```python
from build123d import *

# Parameters (mm, degrees)
SKETCH_1_W               = 100
SKETCH_1_H               = 130
SKETCH_1_R               = 2
EXTRUDE_1_DEPTH          = 2
SKETCH_3_W               = 100
SKETCH_3_H               = 2
EXTRUDE_2_DEPTH          = 45
SKETCH_4_W               = 1.5
SKETCH_4_H               = 110
EXTRUDE_3_DEPTH          = 5
SKETCH_5_W               = 114
SKETCH_5_H               = 47
EXTRUDE_7_DEPTH          = 2
CUT_EXTRUDE_3_DEPTH      = 171.073513517
CUT_EXTRUDE_3_DEPTH_BACK = 171.073513517
EXTRUDE_10_DEPTH         = 1.5
EXTRUDE_11_DEPTH         = 114
CUT_EXTRUDE_4_REACH      = 160.267
SKETCH_13_R              = 2
SKETCH_14_R              = 10
EXTRUDE_12_DEPTH         = 22
CUT_EXTRUDE_5_REACH      = 160.267
SKETCH_15_R              = 1.5
CUT_EXTRUDE_6_REACH      = 176.781
SKETCH_16_R              = 1.5
CUT_EXTRUDE_7_REACH      = 184.153
SKETCH_17_W              = 25
SKETCH_17_H              = 35
CUT_EXTRUDE_8_REACH      = 160.267
SKETCH_18_W              = 20
SKETCH_18_H              = 30
CUT_EXTRUDE_9_REACH      = 176.781
SKETCH_19_W              = 20
SKETCH_19_H              = 28
SKETCH_19_W_2            = 15
CUT_EXTRUDE_10_REACH     = 176.781
SKETCH_20_R              = 3


with BuildPart() as part:
    # 草图1 → 凸台-拉伸1 (new body)
    with BuildSketch(Plane(origin=(0, 0, 0), x_dir=(1, 0, 0), z_dir=(0, 1, 0))):
        with Locations((50, 65)):
            Rectangle(SKETCH_1_W, SKETCH_1_H)
        with Locations(Location((15, 105, 0), (0, 0, 270))):
            Circle(SKETCH_1_R, mode=Mode.SUBTRACT)
        with Locations(Location((15, 19, 0), (0, 0, 270))):
            Circle(SKETCH_1_R, mode=Mode.SUBTRACT)
        with Locations(Location((73, 105, 0), (0, 0, 270))):
            Circle(SKETCH_1_R, mode=Mode.SUBTRACT)
        with Locations(Location((73, 19, 0), (0, 0, 270))):
            Circle(SKETCH_1_R, mode=Mode.SUBTRACT)
    extrude(amount=EXTRUDE_1_DEPTH)

    # 草图3 → 凸台-拉伸2 (add)
    with BuildSketch(Plane(origin=(0, 2, 0), x_dir=(1, 0, 0), z_dir=(0, 1, 0))):
        with Locations((50, 121)):
            Rectangle(SKETCH_3_W, SKETCH_3_H)
        with Locations((50, 9)):
            Rectangle(SKETCH_3_W, SKETCH_3_H)
    extrude(amount=EXTRUDE_2_DEPTH)

    # 草图4 → 凸台-拉伸3 (add)
    with BuildSketch(Plane(origin=(0, 2, 0), x_dir=(1, 0, 0), z_dir=(0, 1, 0))):
        with Locations((91.25, 65)):
            Rectangle(SKETCH_4_W, SKETCH_4_H)
    extrude(amount=EXTRUDE_3_DEPTH)

    # 草图5 → 凸台-拉伸7 (add)
    with BuildSketch(Plane.ZY):
        with Locations((-65, 23.5)):
            Rectangle(SKETCH_5_W, SKETCH_5_H)
    extrude(amount=EXTRUDE_7_DEPTH)

    # 草图6 → 切除-拉伸3 (cut, two sides: drawn at the far end of the back side and taken through both)
    with BuildSketch(Plane(origin=(0, 2, 0), x_dir=(1, 0, 0), z_dir=(0, 1, 0)).offset(-CUT_EXTRUDE_3_DEPTH_BACK)):
        Polygon((0, 8), (92, 8), (92, 122), (0, 122), (0, 130), (100, 130), (100, 117), (100, 13), (100, 0), (0, 0), align=None)
    extrude(amount=CUT_EXTRUDE_3_DEPTH + CUT_EXTRUDE_3_DEPTH_BACK, mode=Mode.SUBTRACT)

    # 草图11 → 凸台-拉伸10 (add)
    with BuildSketch(Plane(origin=(92, 0, 0), x_dir=(0, 0, -1), z_dir=(1, 0, 0))):
        Polygon((8, 47), (122, 47), (122, 42), (122, 0), (110, 0), (110, 37), (16, 37), (16, 0), (8, 0), align=None)
    extrude(amount=-EXTRUDE_10_DEPTH)

    # 草图12 → 凸台-拉伸11 (add, through all)
    with BuildSketch(Plane.XY.offset(-8)):
        with BuildLine():
            Line((91, 47), (91, 48.5))
            ThreePointArc((91, 48.5), (90, 51.796662955), (89, 48.5))
            Line((89, 48.5), (89, 47))
            Line((89, 47), (86, 47))
            Line((86, 47), (86, 45))
            Line((86, 45), (90, 45))
            Line((90, 45), (90, 42.318790087))
            Line((90, 42.318790087), (92, 42.318790087))
            Line((92, 42.318790087), (92, 44))
            Line((92, 44), (93.5, 44))
            ThreePointArc((93.5, 44), (96.796662955, 45), (93.5, 46))
            Line((93.5, 46), (92, 46))
            Line((92, 46), (92, 47))
            Line((92, 47), (91, 47))
        make_face()
        with BuildLine():
            Line((0, 42.318790087), (0, 45))
            Line((0, 45), (4, 45))
            Line((4, 45), (4, 47))
            Line((4, 47), (1, 47))
            Line((1, 47), (1, 48.5))
            ThreePointArc((1, 48.5), (0, 51.796662955), (-1, 48.5))
            Line((-1, 48.5), (-1, 47))
            Line((-1, 47), (-2, 47))
            Line((-2, 47), (-2, 46))
            Line((-2, 46), (-3.5, 46))
            ThreePointArc((-3.5, 46), (-6.796662955, 45), (-3.5, 44))
            Line((-3.5, 44), (-2, 44))
            Line((-2, 44), (-2, 42.318790087))
            Line((-2, 42.318790087), (0, 42.318790087))
        make_face()
        with BuildLine():
            Line((-1, 0), (-1, -1.5))
            ThreePointArc((-1, -1.5), (0, -4.796662955), (1, -1.5))
            Line((1, -1.5), (1, 0))
            Line((1, 0), (4, 0))
            Line((4, 0), (4, 2))
            Line((4, 2), (0, 2))
            Line((0, 2), (0, 4.681209913))
            Line((0, 4.681209913), (-2, 4.681209913))
            Line((-2, 4.681209913), (-2, 3))
            Line((-2, 3), (-3.5, 3))
            ThreePointArc((-3.5, 3), (-6.796662955, 2), (-3.5, 1))
            Line((-3.5, 1), (-2, 1))
            Line((-2, 1), (-2, 0))
            Line((-2, 0), (-1, 0))
        make_face()
        with BuildLine():
            Line((90, 4.681209913), (90, 2))
            Line((90, 2), (86, 2))
            Line((86, 2), (86, 0))
            Line((86, 0), (89, 0))
            Line((89, 0), (89, -1.5))
            ThreePointArc((89, -1.5), (90, -4.796662955), (91, -1.5))
            Line((91, -1.5), (91, 0))
            Line((91, 0), (92, 0))
            Line((92, 0), (92, 1))
            Line((92, 1), (93.5, 1))
            ThreePointArc((93.5, 1), (96.796662955, 2), (93.5, 3))
            Line((93.5, 3), (92, 3))
            Line((92, 3), (92, 4.681209913))
            Line((92, 4.681209913), (90, 4.681209913))
        make_face()
    extrude(amount=-EXTRUDE_11_DEPTH)

    # 草图13 → 切除-拉伸4 (cut, up to next)
    with BuildSketch(Plane.XY.offset(-8), mode=Mode.PRIVATE) as cut_extrude_4_sk1:
        with Locations((86, 40.599475321)):
            Circle(SKETCH_13_R)
    cut_extrude_4_tool1 = extrude(cut_extrude_4_sk1.sketch, amount=-CUT_EXTRUDE_4_REACH, mode=Mode.PRIVATE) & part.part
    # 草图13 → 切除-拉伸4 (cut, up to next)
    with BuildSketch(Plane.XY.offset(-8), mode=Mode.PRIVATE) as cut_extrude_4_sk2:
        with Locations((86, 5.599475321)):
            Circle(SKETCH_13_R)
    cut_extrude_4_tool2 = extrude(cut_extrude_4_sk2.sketch, amount=-CUT_EXTRUDE_4_REACH, mode=Mode.PRIVATE) & part.part
    # 草图13 → 切除-拉伸4 (cut, up to next)
    with BuildSketch(Plane.XY.offset(-8), mode=Mode.PRIVATE) as cut_extrude_4_sk3:
        with Locations((4, 5.599475321)):
            Circle(SKETCH_13_R)
    cut_extrude_4_tool3 = extrude(cut_extrude_4_sk3.sketch, amount=-CUT_EXTRUDE_4_REACH, mode=Mode.PRIVATE) & part.part
    # 草图13 → 切除-拉伸4 (cut, up to next)
    with BuildSketch(Plane.XY.offset(-8), mode=Mode.PRIVATE) as cut_extrude_4_sk4:
        with Locations((4, 40.599475321)):
            Circle(SKETCH_13_R)
    cut_extrude_4_tool4 = extrude(cut_extrude_4_sk4.sketch, amount=-CUT_EXTRUDE_4_REACH, mode=Mode.PRIVATE) & part.part
    add(cut_extrude_4_tool1.solids().sort_by_distance((86, 40.599475, -8))[0], mode=Mode.SUBTRACT)
    add(cut_extrude_4_tool2.solids().sort_by_distance((86, 5.599475, -8))[0], mode=Mode.SUBTRACT)
    add(cut_extrude_4_tool3.solids().sort_by_distance((4, 5.599475, -8))[0], mode=Mode.SUBTRACT)
    add(cut_extrude_4_tool4.solids().sort_by_distance((4, 40.599475, -8))[0], mode=Mode.SUBTRACT)

    # 草图14 → 凸台-拉伸12 (add)
    with BuildSketch(Plane(origin=(0, 0, -122), x_dir=(-1, 0, 0), z_dir=(0, 0, -1))):
        with Locations(Location((-45, 23.5, 0), (0, 0, 180))):
            Circle(SKETCH_14_R)
    extrude(amount=EXTRUDE_12_DEPTH)

    # 草图15 → 切除-拉伸5 (cut, up to next)
    with BuildSketch(Plane(origin=(0, 0, -122), x_dir=(-1, 0, 0), z_dir=(0, 0, -1)), mode=Mode.PRIVATE) as cut_extrude_5_sk1:
        with Locations((-62, 32)):
            Circle(SKETCH_15_R)
    cut_extrude_5_tool1 = extrude(cut_extrude_5_sk1.sketch, amount=-CUT_EXTRUDE_5_REACH, mode=Mode.PRIVATE) & part.part
    # 草图15 → 切除-拉伸5 (cut, up to next)
    with BuildSketch(Plane(origin=(0, 0, -122), x_dir=(-1, 0, 0), z_dir=(0, 0, -1)), mode=Mode.PRIVATE) as cut_extrude_5_sk2:
        with Locations((-62, 15)):
            Circle(SKETCH_15_R)
    cut_extrude_5_tool2 = extrude(cut_extrude_5_sk2.sketch, amount=-CUT_EXTRUDE_5_REACH, mode=Mode.PRIVATE) & part.part
    add(cut_extrude_5_tool1.solids().sort_by_distance((62, 32, -122))[0], mode=Mode.SUBTRACT)
    add(cut_extrude_5_tool2.solids().sort_by_distance((62, 15, -122))[0], mode=Mode.SUBTRACT)

    # 草图16 → 切除-拉伸6 (cut, up to next)
    with BuildSketch(Plane(origin=(0, 0, -144), x_dir=(-1, 0, 0), z_dir=(0, 0, -1)), mode=Mode.PRIVATE) as cut_extrude_6_sk1:
        with Locations((-45, 23.5)):
            Circle(SKETCH_16_R)
    cut_extrude_6_tool1 = extrude(cut_extrude_6_sk1.sketch, amount=-CUT_EXTRUDE_6_REACH, mode=Mode.PRIVATE) & part.part
    add(cut_extrude_6_tool1.solids().sort_by_distance((45, 23.5, -144))[0], mode=Mode.SUBTRACT)

    # 草图17 → 切除-拉伸7 (cut, up to next)
    with BuildSketch(Plane.ZY.offset(2), mode=Mode.PRIVATE) as cut_extrude_7_sk1:
        with Locations((-97.5, 23)):
            Rectangle(SKETCH_17_W, SKETCH_17_H)
    cut_extrude_7_tool1 = extrude(cut_extrude_7_sk1.sketch, amount=-CUT_EXTRUDE_7_REACH, mode=Mode.PRIVATE) & part.part
    # 草图17 → 切除-拉伸7 (cut, up to next)
    with BuildSketch(Plane.ZY.offset(2), mode=Mode.PRIVATE) as cut_extrude_7_sk2:
        with Locations((-62.5, 23)):
            Rectangle(SKETCH_17_W, SKETCH_17_H)
    cut_extrude_7_tool2 = extrude(cut_extrude_7_sk2.sketch, amount=-CUT_EXTRUDE_7_REACH, mode=Mode.PRIVATE) & part.part
    # 草图17 → 切除-拉伸7 (cut, up to next)
    with BuildSketch(Plane.ZY.offset(2), mode=Mode.PRIVATE) as cut_extrude_7_sk3:
        with Locations((-27.5, 23)):
            Rectangle(SKETCH_17_W, SKETCH_17_H)
    cut_extrude_7_tool3 = extrude(cut_extrude_7_sk3.sketch, amount=-CUT_EXTRUDE_7_REACH, mode=Mode.PRIVATE) & part.part
    add(cut_extrude_7_tool1.solids().sort_by_distance((-2, 23, -97.5))[0], mode=Mode.SUBTRACT)
    add(cut_extrude_7_tool2.solids().sort_by_distance((-2, 23, -62.5))[0], mode=Mode.SUBTRACT)
    add(cut_extrude_7_tool3.solids().sort_by_distance((-2, 23, -27.5))[0], mode=Mode.SUBTRACT)

    # 草图18 → 切除-拉伸8 (cut, up to next)
    with BuildSketch(Plane(origin=(0, 0, -122), x_dir=(-1, 0, 0), z_dir=(0, 0, -1)), mode=Mode.PRIVATE) as cut_extrude_8_sk1:
        with Locations((-18, 25)):
            Rectangle(SKETCH_18_W, SKETCH_18_H)
    cut_extrude_8_tool1 = extrude(cut_extrude_8_sk1.sketch, amount=-CUT_EXTRUDE_8_REACH, mode=Mode.PRIVATE) & part.part
    add(cut_extrude_8_tool1.solids().sort_by_distance((18, 25, -122))[0], mode=Mode.SUBTRACT)

    # 草图19 → 切除-拉伸9 (cut, up to next)
    with BuildSketch(Plane.XY.offset(-8), mode=Mode.PRIVATE) as cut_extrude_9_sk1:
        with Locations((18, 23)):
            Rectangle(SKETCH_19_W, SKETCH_19_H)
    cut_extrude_9_tool1 = extrude(cut_extrude_9_sk1.sketch, amount=-CUT_EXTRUDE_9_REACH, mode=Mode.PRIVATE) & part.part
    # 草图19 → 切除-拉伸9 (cut, up to next)
    with BuildSketch(Plane.XY.offset(-8), mode=Mode.PRIVATE) as cut_extrude_9_sk2:
        with Locations((45.5, 23)):
            Rectangle(SKETCH_19_W_2, SKETCH_19_H)
    cut_extrude_9_tool2 = extrude(cut_extrude_9_sk2.sketch, amount=-CUT_EXTRUDE_9_REACH, mode=Mode.PRIVATE) & part.part
    # 草图19 → 切除-拉伸9 (cut, up to next)
    with BuildSketch(Plane.XY.offset(-8), mode=Mode.PRIVATE) as cut_extrude_9_sk3:
        with Locations((73, 23)):
            Rectangle(SKETCH_19_W, SKETCH_19_H)
    cut_extrude_9_tool3 = extrude(cut_extrude_9_sk3.sketch, amount=-CUT_EXTRUDE_9_REACH, mode=Mode.PRIVATE) & part.part
    add(cut_extrude_9_tool1.solids().sort_by_distance((18, 23, -8))[0], mode=Mode.SUBTRACT)
    add(cut_extrude_9_tool2.solids().sort_by_distance((45.5, 23, -8))[0], mode=Mode.SUBTRACT)
    add(cut_extrude_9_tool3.solids().sort_by_distance((73, 23, -8))[0], mode=Mode.SUBTRACT)

    # 草图20 → 切除-拉伸10 (cut, up to next)
    with BuildSketch(Plane(origin=(0, 0, -144), x_dir=(-1, 0, 0), z_dir=(0, 0, -1)), mode=Mode.PRIVATE) as cut_extrude_10_sk1:
        with Locations((-45, 29.5)):
            Circle(SKETCH_20_R)
    cut_extrude_10_tool1 = extrude(cut_extrude_10_sk1.sketch, amount=-CUT_EXTRUDE_10_REACH, mode=Mode.PRIVATE) & part.part
    add(cut_extrude_10_tool1.solids().sort_by_distance((45, 29.5, -144))[0], mode=Mode.SUBTRACT)


solid = part.part
```
Model file for the job. Use its own axes, mm. A direction names the side the tool comes from. Round coordinates to 2 decimals unless told otherwise and drop trailing zeros. Write each loop counter-clockwise with the first axis right and the second up, starting at its lowest first coordinate (ties: lowest second). Pieces come first, ordered by that corner, then holes. Notation, with made-up numbers: (27, -19.75) - (49, -19.75) arc R6 ccw to (49, -9.75) - close; hole circle Ø3 at (52, 11). An arc over 180 degrees is marked (long way). One line per item, written item: value.
(1) Cut at C-C, the plane x = 31. Give the cut face in (y, z), plus the area to 3 significant figures.
Values follow:
outline: (0, -122) - (47, -122) - (47, -120) - (2, -120) - (2, -10) - (47, -10) - (47, -8) - (0, -8) - close
area: 408 mm²
(2) Cut at B-B, the plane z = -19. Give the number of separate pieces and of enclosed holes in the cut face, plus the area to 3 significant figures.
Values follow:
separate pieces: 5
enclosed holes: 0
area: 336 mm²
(3) 3-axis set-ups, long thin cutter, end or side, ignore diameter. For faces 1 (the cylindrical face through (-6.796, 2.064, -64.202)), 2 (the flat face through (88, 45, -64)), 3 (the cylindrical face through (3.74, 42.582, -8.986)): which of +Z, -Z, +X, -X, +Y, -Y reach the whole face in a straight line?
Values follow:
face 1: +Z, -Z
face 2: none
face 3: +Z
(4) Two-plate mould, pull along Y, no slides. Class faces 4 (the cylindrical face through (35.01, 23.06, -132.85)), 5 (the flat face through (56, 24, -8)), 6 (the cylindrical face through (-6.796, 45.064, -64.202)): pulls with the +Y half, pulls with the -Y half, needs draft (parallel to the pull), parting line crosses it, or undercut.
Values follow:
face 4: parting line crosses it
face 5: needs draft
face 6: undercut
(5) Drop flat-ended pins along their axis: P1, Ø1.2, axis at y = -0.5, z = -85, coming from the +X side; P2, Ø10, axis at x = 83.5, z = -44.5, coming from the +Y side; P3, Ø1.6, axis at x = -1, z = -25.5, coming from the -Y side; P4, Ø6, axis at y = 31.5, z = -29.5, coming from the -X side. Give the stop position or say it passes through.
Values follow:
P1: stops at x = 92
P2: stops at y = 50.99
P3: stops at y = -4.79
P4: passes through
(6) Wall check: probe 1 along Y at (x, z) = (4, -8.6); probe 2 along Y at (x, z) = (45, -130); probe 3 along Z at (x, y) = (32, 27). Give the ranges that are in metal, low to high.
Values follow:
probe 1: y = 0 to 3.6, 7.6 to 38.6, 42.6 to 47
probe 2: y = 13.5 to 22, 25 to 26.5, 32.5 to 33.5
probe 3: z = -122 to -120, -10 to -8
(7) Cut at A-A, the plane x = 45. Give the cut face in (y, z).
Values follow:
outline: (0, -122) - (13.5, -122) - (13.5, -144) - (22, -144) - (22, -120) - (2, -120) - (2, -10) - (9, -10) - (9, -8) - (0, -8) - close; (25, -144) - (26.5, -144) - (26.5, -120) - (25, -120) - close; (32.5, -144) - (33.5, -144) - (33.5, -122) - (47, -122) - (47, -120) - (32.5, -120) - close; (37, -10) - (47, -10) - (47, -8) - (37, -8) - close
